Autodesk Inventor part; units mm, degrees
ref_plane "YZ Plane" through (0, 0, 0) normal (1, 0, 0) x (0, 1, 0)
ref_plane "XZ Plane" through (0, 0, 0) normal (0, 1, 0) x (-1, 0, 0)
ref_plane "XY Plane" through (0, 0, 0) normal (0, 0, 1) x (1, 0, 0)
sketch "Sketch1" plane through (0, 0, 0) normal (0, 0, 1) x (1, 0, 0)
  circle A0 centre (0, 0) radius 1.8
  line L0 (-3.25, 3.25) -> (3.25, 3.25)
  line L1 (3.25, 3.25) -> (3.25, -3.25)
  line L2 (3.25, -3.25) -> (-3.25, -3.25)
  line L3 (-3.25, -3.25) -> (-3.25, 3.25)
  point P0 (3.25, 0)
  point P1 (0, 3.25)
  dimension "d0" = 3.6
  dimension "d24" = 6.5
extrude "Extrusion1" add sketch "Sketch1" along normal blind 20
fillet "Fillet3" radius 2 4 edges at (3.25, 3.25, 10) (3.25, -3.25, 10) (-3.25, -3.25, 10) (-3.25, 3.25, 10)
chamfer "Chamfer4" distance 0.4 angle 45 18 edges at (-2.6642, -2.6642, 20) (-3.25, 0, 20) (-2.6642, 2.6642, 20) (0, 3.25, 20) (2.6642, 2.6642, 20) (3.25, 0, 20) (2.6642, -2.6642, 20) (0, -3.25, 20) (2.6642, -2.6642, 0) (3.25, 0, 0) (2.6642, 2.6642, 0) (0, 3.25, 0) (-2.6642, 2.6642, 0) (-3.25, 0, 0) (-2.6642, -2.6642, 0) (0, -3.25, 0) (-1.8, 0, 20) (-1.8, 0, 0)
properties part number "shaft-20mm-squareipt" material "ABS Plastic"
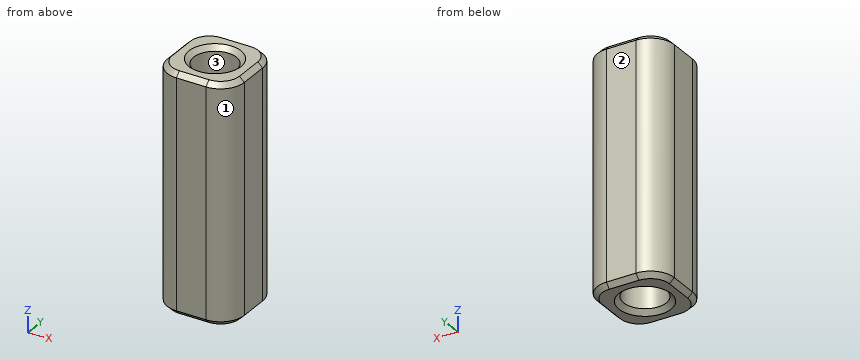
The model under review builds one solid part; all positions refer to its coordinate system, in mm. Face numbers are marked on the shaded views. Round coordinates to 2 decimals unless told otherwise and drop trailing zeros. Loops run counter-clockwise (first coordinate to the right, second up) from the corner with the lowest first, then second, coordinate; pieces in that order, holes last. Notation, with made-up numbers: (-20.75, 31.25) - (10.25, 31.25) arc R22 cw to (10.25, 65.25) - close; hole circle Ø11 at (16, 10). An arc over 180 degrees is marked (long way). Write each question's results on one line, items separated by ' | '. Start each with the question number.
Q1. Draft analysis for pull direction Y (two halves, no side actions). For the marked faces 1, 2 and 3, state which applies: pulls with the +Y half, pulls with the -Y half, needs draft (parallel to the pull), parting line crosses it, or undercut.
Q2. Insertion check: P1, Ø2, axis at x = -2, y = 0.5, coming from the +Z side. The pin has a flat end and moves straight along its axis. Give the tip position at first contact, or say it passes through.
Q3. Take a section at A-A on x = 0. Give the boundary of the cut face in (y, z).
Q4. Wall thickness on line 1 along Y through (x, z) = (0, 5.25); line 2 along X through (y, z) = (1.5, 18.5); line 3 along X through (y, z) = (-1, 18.5): over which ranges is each line inside the solid? List them lowest first. Write a range as [from, to].
Q5. Take a section at B-B on z = 4.75. Give the boundary of the cut face in (x, y), plus the area to 3 significant figures.
Data:
1) face 1: pulls with the -Y half | face 2: pulls with the +Y half | face 3: undercut
2) P1: stops at z = 20
3) outline: (-3.25, 0.4) - (-2.85, 0) - (-2.2, 0) - (-1.8, 0.4) - (-1.8, 19.6) - (-2.2, 20) - (-2.85, 20) - (-3.25, 19.6) - close; (1.8, 0.4) - (2.2, 0) - (2.85, 0) - (3.25, 0.4) - (3.25, 19.6) - (2.85, 20) - (2.2, 20) - (1.8, 19.6) - close
4) line 1: y = [-3.25, -1.8], [1.8, 3.25] | line 2: x = [-3.23, -0.99], [0.99, 3.23] | line 3: x = [-3.25, -1.5], [1.5, 3.25]
5) outline: (-3.25, -1.25) arc R2 ccw to (-1.25, -3.25) - (1.25, -3.25) arc R2 ccw to (3.25, -1.25) - (3.25, 1.25) arc R2 ccw to (1.25, 3.25) - (-1.25, 3.25) arc R2 ccw to (-3.25, 1.25) - close; hole circle Ø3.6 at (0, 0) | area: 28.6 mm²
